Source: CAD feature listing. Evaluate the final solid. Frame: model axes, mm. Face numbers are marked on the shaded views. A direction names the side the tool comes from. Give positions to 0.01 mm unless a question says otherwise; leave off trailing zeros. Order: outer loops, then holes, each group sorted by start corner. A loop starts at its lowest first (then second) coordinate and runs counter-clockwise, first axis right, second up. Notation, with made-up numbers: M -4,76.25 L 54,76.25 A34 ccw 54,112.25 Z; hole C 37,41 d5. An arc over 180 degrees is marked long. Answer as a JSON object with one key per item and string values. Group by question number.
1. Set-up query: the marked faces 1, 2 and 3. Return all of +Z, -Z, +X, -X, +Y, -Y with unobstructed straight access to the full face (end or side cutting, diameter ignored); none if empty.
2. Section query A-A (x = 13.8). Output: boundary loops of the cut face in (y, z).
3. Section query B-B (y = 18.5). Output: boundary loops of the cut face in (x, z).
4. Section query C-C (z = 4.5). Output: boundary loops of the cut face in (x, y), plus the area to 3 significant figures.
5. Section query D-D (x = 0). Output: boundary loops of the cut face in (y, z), plus the area to 3 significant figures.
6. Pin query (flat end, axial travel): P1, Ø1, axis at x = 12.5, y = 15.5, coming from the -Z side; P2, Ø5, axis at y = 22.5, z = -1.5, coming from the -X side; P3, Ø3.5, axis at x = 13, z = 2, coming from the +Y side; P4, Ø3.5, axis at y = 23, z = -1.5, coming from the +X side. Return the tip coordinate at first contact, or that it passes through.
7. Material intervals for L1, parallel to Z at x = 13.8, y = 17.6; L2, parallel to X at y = 17.7, z = 0; L3, parallel to X at y = 3, z = 1.5, sorted ascending. Write a range as [from, to].
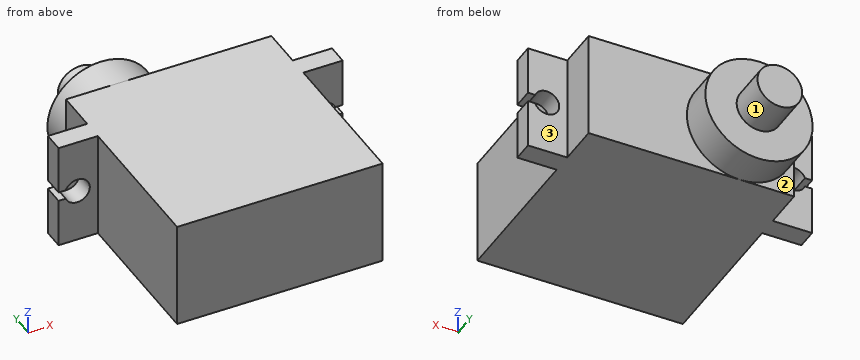
from build123d import *

# Parameters (mm, degrees)
CROQUIS1_W              = 23
CROQUIS1_H              = 12
SALIENTE_EXTRUIR1_DEPTH = 24
CROQUIS2_W              = 12
CROQUIS2_H              = 2.3
SALIENTE_EXTRUIR2_DEPTH = 4.4
CORTAR_EXTRUIR1_REACH   = 27.791
CROQUIS4_R              = 6
SALIENTE_EXTRUIR4_DEPTH = 4
CROQUIS5_R              = 2.5
SALIENTE_EXTRUIR5_DEPTH = 4.5


with BuildPart() as part:
    # Croquis1 → Saliente-Extruir1 (new body)
    with BuildSketch(Plane(origin=(0, 0, 0), x_dir=(1, 0, 0), z_dir=(0, 1, 0))):
        Rectangle(CROQUIS1_W, CROQUIS1_H)
    extrude(amount=SALIENTE_EXTRUIR1_DEPTH)

    # Croquis2 → Saliente-Extruir2 (add)
    with BuildSketch(Plane.ZY.offset(11.5)):
        with Locations((0, 18.25)):
            Rectangle(CROQUIS2_W, CROQUIS2_H)
    saliente_extruir2 = extrude(amount=SALIENTE_EXTRUIR2_DEPTH)

    # Croquis3 → Cortar-Extruir1 (cut, up to next)
    with BuildSketch(Plane(origin=(0, 19.4, 0), x_dir=(1, 0, 0), z_dir=(0, 1, 0)), mode=Mode.PRIVATE) as cortar_extruir1_sk1:
        with BuildLine():
            Line((-15.101550129, -0.515720139), (-15.9, -0.515720139))
            Line((-15.9, -0.515720139), (-15.9, 0.515720139))
            Line((-15.9, 0.515720139), (-15.101550129, 0.515720139))
            ThreePointArc((-15.101550129, 0.515720139), (-12.4, 0), (-15.101550129, -0.515720139))
        make_face()
    cortar_extruir1_tool1 = extrude(cortar_extruir1_sk1.sketch, amount=-CORTAR_EXTRUIR1_REACH, mode=Mode.PRIVATE) & part.part
    cortar_extruir1 = cortar_extruir1_tool1.solids().sort_by_distance((-13.989391, 19.4, 0))[0]
    add(cortar_extruir1, mode=Mode.SUBTRACT)

    # Simetría1: Saliente-Extruir2, Cortar-Extruir1 across plane
    add(saliente_extruir2.mirror(Plane(origin=(0, 0, 0), x_dir=(0, 0, 1), z_dir=(1, 0, 0))))
    add(cortar_extruir1.mirror(Plane(origin=(0, 0, 0), x_dir=(0, 0, 1), z_dir=(1, 0, 0))), mode=Mode.SUBTRACT)

    # Croquis4 → Saliente-Extruir4 (add)
    with BuildSketch(Plane(origin=(0, 24, 0), x_dir=(1, 0, 0), z_dir=(0, 1, 0))):
        with Locations(Location((-5.5, 0, 0), (0, 0, 270))):
            Circle(CROQUIS4_R)
    extrude(amount=SALIENTE_EXTRUIR4_DEPTH)

    # Croquis5 → Saliente-Extruir5 (add)
    with BuildSketch(Plane(origin=(0, 28, 0), x_dir=(1, 0, 0), z_dir=(0, 1, 0))):
        with Locations(Location((-5.5, 0, 0), (0, 0, 270))):
            Circle(CROQUIS5_R)
    extrude(amount=SALIENTE_EXTRUIR5_DEPTH)


solid = part.part
Answer sheet:
{
 "1": {"face 1": "+Y", "face 2": "-Z, -X, +Y", "face 3": "+Z, -Z, +X, +Y"},
 "2": {"outline": "M 17.1,-6 L 19.4,-6 L 19.4,-1.4 L 17.1,-1.4 Z; M 17.1,1.4 L 19.4,1.4 L 19.4,6 L 17.1,6 Z"},
 "3": {"outline": "M -15.9,-6 L 15.9,-6 L 15.9,-0.52 L 15.1,-0.52 A1.4 cw long 15.1,0.52 L 15.9,0.52 L 15.9,6 L -15.9,6 L -15.9,0.52 L -15.1,0.52 A1.4 cw long -15.1,-0.52 L -15.9,-0.52 Z"},
 "4": {"outline": "M -15.9,17.1 L -11.5,17.1 L -11.5,0 L 11.5,0 L 11.5,17.1 L 15.9,17.1 L 15.9,19.4 L 11.5,19.4 L 11.5,24 L -1.53,24 L -1.53,28 L -9.47,28 L -9.47,24 L -11.5,24 L -11.5,19.4 L -15.9,19.4 Z", "area": "604 mm^2"},
 "5": {"outline": "M 0,-6 L 24,-6 L 24,-2.4 L 28,-2.4 L 28,2.4 L 24,2.4 L 24,6 L 0,6 Z", "area": "307 mm^2"},
 "6": {"P1": "through", "P2": "x = -11.5", "P3": "y = 24", "P4": "x = 11.5"},
 "7": {"L1": "[-6, -1.4], [1.4, 6]", "L2": "[-12.4, 12.4]", "L3": "[-11.5, 11.5]"}
}
